```python
from build123d import *

# Parameters (mm, degrees)
EXTRUDE_1_DEPTH     = 13
SKETCH_2_OUTSIDE_W  = 38.11
SKETCH_2_OUTSIDE_H  = 37.182
SKETCH_2_OUTSIDE_R  = 0.75
CUT_EXTRUDE_1_DEPTH = 13
CUT_EXTRUDE_1_TAPER = 45
SKETCH_3_OUTSIDE_W  = 12.11
SKETCH_3_OUTSIDE_H  = 11.182
SKETCH_3_OUTSIDE_R  = 2.35
CUT_EXTRUDE_2_DEPTH = 5
SKETCH_4_R          = 1
CUT_EXTRUDE_3_DEPTH = 12
SKETCH_5_R          = 0.15
CUT_EXTRUDE_4_DEPTH = 1
SKETCH_6_R          = 2.9
SKETCH_6_R_2        = 2.35
EXTRUDE_2_DEPTH     = 4
CHAMFER_1_SIZE      = 0.3


with BuildPart() as part:
    # Эскиз1 → Бобышка-Вытянуть1 (new body)
    with BuildSketch(Plane.XY):
        Polygon((3.464101615, 0), (1.732050808, 3), (-1.732050808, 3), (-3.464101615, 0), (-1.732050808, -3), (1.732050808, -3), align=None)
    extrude(amount=EXTRUDE_1_DEPTH)

    # Эскиз2 outside → Вырез-Вытянуть1 (cut)
    with BuildSketch(Plane.XY.offset(13)):
        Rectangle(SKETCH_2_OUTSIDE_W, SKETCH_2_OUTSIDE_H)
        Circle(SKETCH_2_OUTSIDE_R, mode=Mode.SUBTRACT)
    extrude(amount=-CUT_EXTRUDE_1_DEPTH, taper=CUT_EXTRUDE_1_TAPER, mode=Mode.SUBTRACT)

    # Эскиз3 outside → Вырез-Вытянуть2 (cut)
    with BuildSketch(Plane(origin=(0, 0, 0), x_dir=(-1, 0, 0), z_dir=(0, 0, -1))):
        Rectangle(SKETCH_3_OUTSIDE_W, SKETCH_3_OUTSIDE_H)
        Circle(SKETCH_3_OUTSIDE_R, mode=Mode.SUBTRACT)
    extrude(amount=-CUT_EXTRUDE_2_DEPTH, mode=Mode.SUBTRACT)

    # Эскиз4 → Вырез-Вытянуть3 (cut)
    with BuildSketch(Plane(origin=(0, 0, 0), x_dir=(-1, 0, 0), z_dir=(0, 0, -1))):
        Circle(SKETCH_4_R)
    extrude(amount=-CUT_EXTRUDE_3_DEPTH, mode=Mode.SUBTRACT)

    # Эскиз5 → Вырез-Вытянуть4 (cut)
    with BuildSketch(Plane.XY.offset(13)):
        Circle(SKETCH_5_R)
    extrude(amount=-CUT_EXTRUDE_4_DEPTH, mode=Mode.SUBTRACT)

    # Эскиз6 → Бобышка-Вытянуть2 (add)
    with BuildSketch(Plane(origin=(0, 0, 0), x_dir=(-1, 0, 0), z_dir=(0, 0, -1))):
        Circle(SKETCH_6_R)
        Circle(SKETCH_6_R_2, mode=Mode.SUBTRACT)
    extrude(amount=-EXTRUDE_2_DEPTH)

    # Фаска1
    chamfer_1_edges = [part.edges().sort_by_distance(p)[0] for p in [
        (1, 0, 0),
        (2.9, 0, 4),
        (2.9, 0, 0),
    ]]
    chamfer(chamfer_1_edges, length=CHAMFER_1_SIZE)


solid = part.part
```
Build history of the part. All positions in model axes, mm. A direction names the side the tool comes from. Give positions to 0.01 mm unless a question says otherwise; leave off trailing zeros. Loops run counter-clockwise (first coordinate to the right, second up) from the corner with the lowest first, then second, coordinate; pieces in that order, holes last.
Item 1: Drill centre lines: line 1 (Y direction, x = 0, z = 6); line 2 (X direction, y = -1.5, z = 8); line 3 (Y direction, x = 0, z = 12.75). Where is each one in solid material? Low to high.
Answers follow:
line 1: y = -3 to -1, 1 to 3
line 2: x = -2.6 to 2.6
line 3: y = -1 to -0.15, 0.15 to 1
Item 2: Slice it at A-A, the plane x = 0. List the corners of the cut face in (y, z).
Answers follow:
outline: (-3, 5) - (-2.35, 5) - (-2.35, 4) - (-2.6, 4) - (-2.9, 3.7) - (-2.9, 0.3) - (-2.6, 0) - (-1.3, 0) - (-1, 0.3) - (-1, 12) - (-0.15, 12) - (-0.15, 13) - (-0.75, 13) - (-3, 10.75) - close; (0.15, 12) - (1, 12) - (1, 0.3) - (1.3, 0) - (2.6, 0) - (2.9, 0.3) - (2.9, 3.7) - (2.6, 4) - (2.35, 4) - (2.35, 5) - (3, 5) - (3, 10.75) - (0.75, 13) - (0.15, 13) - close
Item 3: Slice it at C-C, the plane z = 11. List the corners of the cut face in (x, y).
Answers follow:
outline: circle Ø5.5 at (0, 0); hole circle Ø2 at (0, 0)
Item 4: Slice it at B-B, the plane z = 5.75. List the corners of the cut face in (x, y), and give its area (3 significant figures).
Answers follow:
outline: (-3.46, 0) - (-1.73, -3) - (1.73, -3) - (3.46, 0) - (1.73, 3) - (-1.73, 3) - close; hole circle Ø2 at (0, 0)
area: 28.0 mm2
Item 5: Which spindle directions (+Z, -Z, +X, -X, +Y, -Y) get a long thin tool onto all of the face, cutting with end or side? Do faces 4 (the face through (-2, -2, 5)), 5 (the face through (0, -1, 6)), 6 (the face through (0, 3, 8)). Say none if no direction does.
Answers follow:
face 4: none
face 5: -Z
face 6: +Z, -Z, +X, -X, +Y
Item 6: Pull direction X, two halves, no side cores. Call faces 1 (the face through (-0.21, 0.24, 12)), 2 (the face through (-2.6, 1.5, 7.8)), 3 (the face through (2.9, 0.1, 2)): released by +X, released by -X, zero draft, split by the parting line, or undercut.
Answers follow:
face 1: undercut
face 2: released by -X
face 3: split by the parting line
Item 7: Flat gauge pin, fed straight in: pin 1 (1 mm diameter, centred on x = -0.5, y = -0.5, fed in from -Z). Where does the tip first touch, or does it go through?
Answers follow:
pin 1: stops at z = 0.09
